The listing builds one solid part. Answer for the finished solid, in the listing's coordinates (mm). Round coordinates to 2 decimals unless told otherwise and drop trailing zeros. Write each loop counter-clockwise with the first axis right and the second up, starting at its lowest first coordinate (ties: lowest second). Pieces come first, ordered by that corner, then holes. Notation, with made-up numbers: (89, 10.5) - (111, 10.5) arc R31 ccw to (111, 36.5) - close; hole circle Ø3 at (72.25, 7). An arc over 180 degrees is marked (long way). Return JSON: item names as keys, results as strings. Group by question number.
from build123d import *

# Parameters (mm, degrees)
CROQUIS1_R              = 4
CROQUIS1_R_2            = 2
SALIENTE_EXTRUIR1_DEPTH = 6
CHAFL_N1_SIZE           = 0.1


with BuildPart() as part:
    # Croquis1 → Saliente-Extruir1 (new body)
    with BuildSketch(Plane.XY):
        Circle(CROQUIS1_R)
        Circle(CROQUIS1_R_2, mode=Mode.SUBTRACT)
    extrude(amount=SALIENTE_EXTRUIR1_DEPTH)

    # Chaflán1
    chafl_n1_edges = [part.edges().sort_by_distance(p)[0] for p in [
        (-4, 0, 0),
        (-4, 0, 6),
        (-2, 0, 0),
        (-2, 0, 6),
    ]]
    chamfer(chafl_n1_edges, length=CHAFL_N1_SIZE)


solid = part.part
(1) Determine the mould class of faces 1 (the cylindrical face through (-0.867, -3.905, 2.959)), 2 (the cylindrical face through (0, -2, 3)), 3 (the flat face through (2, -2, 0)) for opening direction X: +X half, -X half, draft (parallel to the pull), parting line (faces both ways), or undercut.
(2) Consider line 1 (Y direction, x = 0, z = 4.15); line 2 (X direction, y = -0.5, z = 2.6); line 3 (X direction, y = 1, z = 0.35). Determine where each line is inside the solid, lowest interval first.
(3) Find section A-A (x = 0). Write down the section's boundary in (y, z).
(4) Find section C-C (z = 3.95). Write down the section's boundary in (x, y).
(5) A flat-ended cylindrical pin translates along its axis: pin 1 (2 mm diameter, centred on x = -1.5, z = 4.5, fed in from -Y). Find the tip coordinate at first contact, or state that the pin passes through.
Check sheet entries:
{
 "1": {"face 1": "parting line", "face 2": "undercut", "face 3": "draft"},
 "2": {"line 1": "y = -4 to -2, 2 to 4", "line 2": "x = -3.97 to -1.94, 1.94 to 3.97", "line 3": "x = -3.87 to -1.73, 1.73 to 3.87"},
 "3": {"outline": "(-4, 0.1) - (-3.9, 0) - (-2.1, 0) - (-2, 0.1) - (-2, 5.9) - (-2.1, 6) - (-3.9, 6) - (-4, 5.9) - close; (2, 0.1) - (2.1, 0) - (3.9, 0) - (4, 0.1) - (4, 5.9) - (3.9, 6) - (2.1, 6) - (2, 5.9) - close"},
 "4": {"outline": "circle Ø8 at (0, 0); hole circle Ø4 at (0, 0)"},
 "5": {"pin 1": "stops at y = -3.97"}
}
